```python
from build123d import *

# Parameters (mm, degrees)
SKETCH1_W             = 10
SKETCH1_H             = 35
BOSS_EXTRUDE1_DEPTH   = 3
BOSS_EXTRUDE1_2_DEPTH = 3
SKETCH1_3_W           = 10
SKETCH1_3_H           = 5
BOSS_EXTRUDE2_DEPTH   = 31
SKETCH7_W             = 52
SKETCH7_H             = 40
BOSS_EXTRUDE3_DEPTH   = 3
SKETCH8_R             = 12
SKETCH8_R_2           = 2.25
CUT_EXTRUDE4_DEPTH    = 3
SKETCH10_R            = 1.75
CUT_EXTRUDE5_DEPTH    = 3
SKETCH11_W            = 10
SKETCH11_H            = 5
BOSS_EXTRUDE4_DEPTH   = 28


with BuildPart() as part:
    # Sketch1 → Boss-Extrude1 (new body)
    with BuildSketch(Plane(origin=(0, 0, 0), x_dir=(1, 0, 0), z_dir=(0, 1, 0))):
        with Locations((21, 0)):
            Rectangle(SKETCH1_W, SKETCH1_H)
    extrude(amount=BOSS_EXTRUDE1_DEPTH)


with BuildPart() as body_2:
    # Sketch1 → Boss-Extrude1 2 (new body)
    with BuildSketch(Plane(origin=(0, 0, 0), x_dir=(1, 0, 0), z_dir=(0, 1, 0))):
        with Locations((-21, 0)):
            Rectangle(SKETCH1_W, SKETCH1_H)
    extrude(amount=BOSS_EXTRUDE1_2_DEPTH)

    # Sketch1<3> → Boss-Extrude2 (add)
    with BuildSketch(Plane(origin=(0, 0, 0), x_dir=(1, 0, 0), z_dir=(0, 1, 0))):
        with Locations((-21, 20)):
            Rectangle(SKETCH1_3_W, SKETCH1_3_H)
        with Locations((21, 20)):
            Rectangle(SKETCH1_3_W, SKETCH1_3_H)
    extrude(amount=BOSS_EXTRUDE2_DEPTH)

    # Sketch7 → Boss-Extrude3 (add)
    with BuildSketch(Plane(origin=(0, 31, 0), x_dir=(1, 0, 0), z_dir=(0, 1, 0))):
        with Locations((0, 2.5)):
            Rectangle(SKETCH7_W, SKETCH7_H)
    extrude(amount=BOSS_EXTRUDE3_DEPTH)

    # Sketch8 → Cut-Extrude4 (cut)
    with BuildSketch(Plane(origin=(0, 34, 0), x_dir=(1, 0, 0), z_dir=(0, 1, 0))):
        with Locations((4, 0.5)):
            Circle(SKETCH8_R)
        with Locations((-6, -11.5)):
            Circle(SKETCH8_R_2)
        with Locations((14, 12.5)):
            Circle(SKETCH8_R_2)
    extrude(amount=-CUT_EXTRUDE4_DEPTH, mode=Mode.SUBTRACT)


with BuildPart() as cut_extrude5_tool:
    # Sketch10 → Cut-Extrude5 (new body)
    with BuildSketch(Plane(origin=(0, 3, 0), x_dir=(1, 0, 0), z_dir=(0, 1, 0))):
        with Locations((-19, 0)):
            Circle(SKETCH10_R)
        with Locations((19, 0)):
            Circle(SKETCH10_R)
    extrude(amount=-CUT_EXTRUDE5_DEPTH)


with BuildPart() as part_1:
    add(part.part)

    # Cut-Extrude5: cut by cut_extrude5_tool
    add(cut_extrude5_tool.part, mode=Mode.SUBTRACT)



with BuildPart() as body_2_1:
    add(body_2.part)

    # Cut-Extrude5: cut by cut_extrude5_tool
    add(cut_extrude5_tool.part, mode=Mode.SUBTRACT)


with BuildPart() as part_2:
    add(part_1.part)

    add(body_2_1.part)  # Boss-Extrude4 merges body 2
    # Sketch11 → Boss-Extrude4 (add)
    with BuildSketch(Plane(origin=(0, 3, 0), x_dir=(1, 0, 0), z_dir=(0, 1, 0))):
        with Locations((-21, -15)):
            Rectangle(SKETCH11_W, SKETCH11_H)
        with Locations((21, -15)):
            Rectangle(SKETCH11_W, SKETCH11_H)
    extrude(amount=BOSS_EXTRUDE4_DEPTH)


solid = part_2.part
```
Work out the finished part from the listing and answer in its coordinate system (mm). A direction names the side the tool comes from. Coordinates: 2 decimals unless noted, no trailing zeros. Loops run counter-clockwise (first coordinate to the right, second up) from the corner with the lowest first, then second, coordinate; pieces in that order, holes last.
1) Section A-A (z = -16) is taken. Give the vertices of the cut face in (x, y), plus the area to 3 significant figures.
Results:
outline: (-26, 0) - (-16, 0) - (-16, 3) - (-26, 3) - close; (-26, 31) - (26, 31) - (26, 34) - (-26, 34) - close; (16, 0) - (26, 0) - (26, 3) - (16, 3) - close
area: 216 mm2
2) Flat-ended cylindrical pins translate along their axes: pin 1 (12 mm diameter, centred on x = -4.5, y = 20.5, fed in from +Z); pin 2 (3 mm diameter, centred on x = 19, z = 0, fed in from -Y). Find the tip coordinate at first contact, or state that the pin passes through.
Results:
pin 1: passes through
pin 2: stops at y = 31
3) Consider probe 1 along X at (y, z) = (1, 0); probe 2 along X at (y, z) = (33, 0); probe 3 along Z at (x, y) = (-6, 32.1). Determine where each line is inside the solid, lowest interval first.
Results:
probe 1: x = -26 to -20.75, -17.25 to -16, 16 to 17.25, 20.75 to 26
probe 2: x = -26 to -7.99, 15.99 to 26
probe 3: z = -22.5 to -7.13, 6.13 to 9.25, 13.75 to 17.5
4) Section C-C (y = 27.5) is taken. Give the vertices of the cut face in (x, z), plus the area to 3 significant figures.
Results:
outline: (-26, -22.5) - (-16, -22.5) - (-16, -17.5) - (-26, -17.5) - close; (-26, 12.5) - (-16, 12.5) - (-16, 17.5) - (-26, 17.5) - close; (16, -22.5) - (26, -22.5) - (26, -17.5) - (16, -17.5) - close; (16, 12.5) - (26, 12.5) - (26, 17.5) - (16, 17.5) - close
area: 200 mm2
5) Section D-D (x = 19) is taken. Give the vertices of the cut face in (y, z), plus the area to 4 significant figures.
Results:
outline: (0, -22.5) - (34, -22.5) - (34, 17.5) - (0, 17.5) - (0, 1.75) - (3, 1.75) - (3, 12.5) - (31, 12.5) - (31, -17.5) - (3, -17.5) - (3, -1.75) - (0, -1.75) - close
area: 509.5 mm2
6) Section B-B (x = 4) is taken. Give the vertices of the cut face in (y, z).
Results:
outline: (31, -22.5) - (34, -22.5) - (34, -12.5) - (31, -12.5) - close; (31, 11.5) - (34, 11.5) - (34, 17.5) - (31, 17.5) - close
7) For faces 4 (the flat face through (-21, 17, -17.5)), 5 (the cylindrical face through (15.21, 32.521, -14.397)), 6 (the flat face through (-16, 2.8, -0.9)), 7 (the cylindrical face through (17.25, 1.52, -0.08)), determine the directions among +Z, -Z, +X, -X, +Y, -Y from which every point of the face is accessible in a straight line to the end or side of a thin tool.
Results:
face 4: +X, -X
face 5: +Y
face 6: +Z, -Z, -Y
face 7: -Y
8) For a pull along Y with two mould halves and no side action, classify faces 1 (the flat face through (-21, 0, -3)), 2 (the flat face through (21, 3, -3)), 3 (the flat face through (26, 2, -2)) as +Y half, -Y half, draft (parallel to the pull), parting line (faces both ways), or undercut.
Results:
face 1: -Y half
face 2: undercut
face 3: draft
